Read the model definition and answer for the solid it produces. Units are mm, in the model's axes. Face numbers are marked on the shaded views. Give positions to 0.01 mm unless a question says otherwise; leave off trailing zeros. Write each loop counter-clockwise with the first axis right and the second up, starting at its lowest first coordinate (ties: lowest second). Pieces come first, ordered by that corner, then holes. Notation, with made-up numbers: (-30.5, 38.5) - (2.5, 38.5) arc R19 ccw to (2.5, 68.5) - close; hole circle Ø9 at (32.5, -11.5). An arc over 180 degrees is marked (long way). Answer as a JSON object with one key per item and string values. Group by question number.
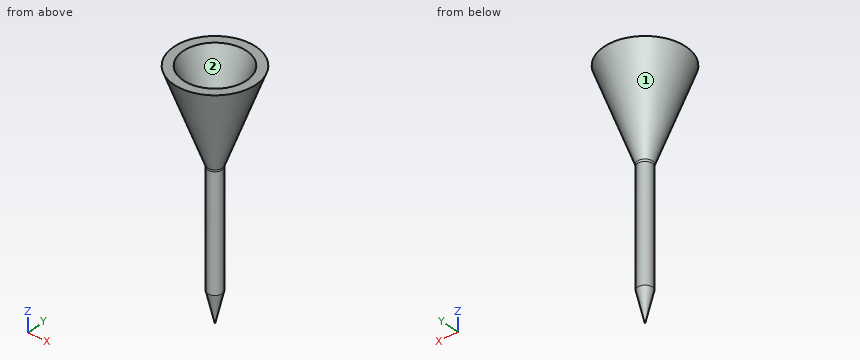
```python
from build123d import *

# Parameters (mm, degrees)
FILLET1_R = 1


with BuildPart() as part:
    # Sketch1 → Revolve1 (revolve)
    with BuildSketch(Plane(origin=(0, 0, 0), x_dir=(0, 0, -1), z_dir=(1, 0, 0)), mode=Mode.PRIVATE) as revolve1_sk:
        Polygon((0, 0), (-4.376068376, 0), (-10, 2.05625), (-16, 4.25), (-16, 5.85), align=None)
        Polygon((-10, 0), (-4.376068376, 0), (-10, 2.05625), align=None)
        Polygon((20, 0), (0, 0), (-4.376068376, 0), (-10, 0), (-10, -1.25), (20, -1.25), align=None)
        Polygon((25.4, -1.25), (20, -1.25), (20, 0), align=None)
    revolve(revolve1_sk.sketch.rotate(Axis((0, -1.25, 10), (0, 0, -1)), 180), axis=Axis((0, -1.25, 10), (0, 0, -1)))

    # Fillet1
    fillet1_edges = [part.edges().sort_by_distance(p)[0] for p in [
        (0, 0, 0),
    ]]
    fillet(fillet1_edges, radius=FILLET1_R)


solid = part.part
```
1) Flat-ended cylindrical pins translate along their axes: pin 1 Ø8 at (y, z) = (-5, -7.5) entering from +X; pin 2 Ø1 at (y, z) = (-2.5, -16) entering from -X; pin 3 Ø1.5 at (x, z) = (5, 3) entering from +Y. Find the tip coordinate at first contact, or state that the pin passes through.
2) Find the intervals of material crossed by line 1 (X direction, y = -5.75, z = 14.5); line 2 (Y direction, x = 0.5, z = 1); line 3 (Z direction, x = 5.5, y = -4.25), in increasing order. Write a range as [from, to].
3) Find section A-A, the plane z = -4. Write down the section's boundary in (x, y).
4) For a pull along X with two mould halves and no side action, classify the marked faces 1 and 2 as released by +X, released by -X, zero draft, split by the parting line, or undercut.
5) Find section B-B, the plane z = 7.5. Write down the section's boundary in (x, y).
Values follow:
{
 "1": {"pin 1": "stops at x = 1.25", "pin 2": "stops at x = -1", "pin 3": "passes through"},
 "2": {"line 1": "x = [-4.76, -2.07], [2.07, 4.76]", "line 2": "y = [-2.79, 0.29]", "line 3": "z = [13.72, 16]"},
 "3": {"outline": "circle Ø2.5 at (0, -1.25)"},
 "4": {"face 1": "split by the parting line", "face 2": "undercut"},
 "5": {"outline": "circle Ø7.98 at (0, -1.25)"}
}
